```python
from build123d import *

# Parameters (mm, degrees)
EXTRUDE_1_DEPTH          = 2.5
SKETCH_5_R               = 0.6
CUT_EXTRUDE_1_DEPTH      = 19.036421485
CUT_EXTRUDE_START        = -2
SKETCH_5_3_R             = 1
CUT_EXTRUDE_2_DEPTH      = 1
REVOLVE_1_ANGLE          = 1
SKETCH_9_R               = 0.6
CUT_EXTRUDE_3_DEPTH      = 41.426698916
SKETCH_9_3_R             = 1
CUT_EXTRUDE_4_DEPTH      = 1
CUT_EXTRUDE_9_DEPTH      = 41.426698916
CUT_EXTRUDE_9_DEPTH_BACK = 41.426698916


with BuildPart() as part:
    # 草图4 → 凸台-拉伸1 (new body)
    with BuildSketch(Plane.XY):
        Polygon((8.5, -1.5), (17.75, -1.5), (17.75, -3.5), (-4.5, -3.5), (-4.5, -1.5), (-0.5, 0), (0, 0), (0, -1.5), (4, -1.5), (4, 0), (4.5, 0), align=None)
    extrude(amount=EXTRUDE_1_DEPTH)

    # 草图5 → 切除-拉伸1 (cut, through all)
    with BuildSketch(Plane(origin=(0, -1.5, 0), x_dir=(1, 0, 0), z_dir=(0, 1, 0))):
        with Locations(Location((2, -1.25, 0), (0, 0, 270))):
            Circle(SKETCH_5_R)
    extrude(amount=-CUT_EXTRUDE_1_DEPTH, mode=Mode.SUBTRACT)

    # 草图5<3> → 切除-拉伸2 (cut)
    with BuildSketch(Plane(origin=(0, -1.5, 0), x_dir=(1, 0, 0), z_dir=(0, 1, 0)).offset(CUT_EXTRUDE_START)):
        with Locations((2, -1.25)):
            Circle(SKETCH_5_3_R)
    extrude(amount=CUT_EXTRUDE_2_DEPTH, mode=Mode.SUBTRACT)

    # 镜向1: part across plane


with BuildPart() as part_1:
    add(part.part)
    add(part.part.mirror(Plane(origin=(17.75, 0, 2.5), x_dir=(0, 0, 1), z_dir=(1, 0, 0))))

    # 草图6 → 旋转1 (revolve)
    with BuildSketch(Plane.XY.offset(2.5)):
        Polygon((0, 0), (-0.5, 0), (-4.5, -1.5), (-4.5, -3.5), (40, -3.5), (40, -1.5), (36, 0), (35.5, 0), (35.5, -1.5), (31.5, -1.5), (31.5, 0), (31, 0), (27, -1.5), (8.5, -1.5), (4.5, 0), (4, 0), (4, -1.5), (0, -1.5), align=None)
    revolve(axis=Axis((-132.25, 94.8535776, 2.5), (0, -1, 0)), revolution_arc=REVOLVE_1_ANGLE)

    # 草图9 → 切除-拉伸3 (cut, through all)
    with BuildSketch(Plane(origin=(0, -1.5, 0), x_dir=(1, 0, 0), z_dir=(0, 1, 0))):
        with Locations(Location((1.994888171, -3.671537391, 0), (0, 0, 180))):
            Circle(SKETCH_9_R)
        with Locations(Location((33.493688748, -3.946423259, 0), (0, 0, 180))):
            Circle(SKETCH_9_R)
    extrude(amount=-CUT_EXTRUDE_3_DEPTH, mode=Mode.SUBTRACT)

    # 草图9<3> → 切除-拉伸4 (cut)
    with BuildSketch(Plane(origin=(0, -1.5, 0), x_dir=(1, 0, 0), z_dir=(0, 1, 0)).offset(CUT_EXTRUDE_START)):
        with Locations((1.994888171, -3.671537391)):
            Circle(SKETCH_9_3_R)
        with Locations((33.493688748, -3.946423259)):
            Circle(SKETCH_9_3_R)
    extrude(amount=CUT_EXTRUDE_4_DEPTH, mode=Mode.SUBTRACT)

    # 草图10 → 切除-拉伸9 (cut, two sides: drawn at the far end of the back side and taken through both)
    with BuildSketch(Plane(origin=(0, -1.5, 0), x_dir=(1, 0, 0), z_dir=(0, 1, 0)).offset(-CUT_EXTRUDE_9_DEPTH_BACK)):
        Polygon((27, -2.5), (27, -1.5), (24.5, -1.5), (25.667850814, -3.5), (20.832149186, -3.5), (22, -1.5), (17.164298372, -1.5), (18.332149186, -3.5), (13.496447557, -3.5), (14.664298372, -1.5), (9.828596743, -1.5), (10.996447557, -3.5), (8.496447557, -3.5), (8.5, -2.5), (-4.5, -2.5), (-4.5, 0), (40, 0), (40, -2.5), align=None)
    extrude(amount=CUT_EXTRUDE_9_DEPTH + CUT_EXTRUDE_9_DEPTH_BACK, mode=Mode.SUBTRACT)


solid = part_1.part
```
The model under review builds one solid part; all positions refer to its coordinate system, in mm. A direction names the side the tool comes from. Round coordinates to 2 decimals unless told otherwise and drop trailing zeros. Loops run counter-clockwise (first coordinate to the right, second up) from the corner with the lowest first, then second, coordinate; pieces in that order, holes last. Notation, with made-up numbers: (16, -13) - (58, -13) arc R14 ccw to (58, -7) - close; hole circle Ø11 at (58.25, 66). An arc over 180 degrees is marked (long way). Write each question's results on one line, items separated by ' | '. Start each with the question number.
Q1. Wall thickness on line 1 along X through (y, z) = (-2.75, 2.1); line 2 along X through (y, z) = (-1.7, 2.55); line 3 along Y through (x, z) = (23.5, 4.35): over which ranges is each line inside the solid? List them lowest first. Write a range as [from, to].
Q2. Tool access review of faces 1 (the flat face through (17.74, -2.514, 2.486)), 2 (the flat face through (2, -2, 2.5)), 3 (the flat face through (34, -2, 2.5)): name each direction out of +Z, -Z, +X, -X, +Y, -Y from which nothing blocks a thin tool from reaching the whole face with its end or side.
Q3. Take a section at C-C on y = -3. Give the boundary of the cut face in (x, z), plus the area to 3 significant figures.
Q4. Draft analysis for pull direction X (two halves, no side actions). For faces 4 (the flat face through (10, -3, 3.5)), 5 (the flat face through (2, -1.5, 4.5)), 6 (the cylindrical face through (39.994, -2.486, 3.982)), 7 (the flat face through (18, -3.5, 4)), state which applies: pulls with the +X half, pulls with the -X half, needs draft (parallel to the pull), parting line crosses it, or undercut.
Q5. Take a section at D-D on x = 35. Give the boundary of the cut face in (y, z).
Q6. Insertion check: P1, Ø1, axis at x = 16, y = -3, coming from the -Z side; P2, Ø0.5, axis at y = -3, z = 2, coming from the +X side; P3, Ø1.9, axis at x = 33.49, z = 3.95, coming from the -Y side. Each pin has a flat end and moves straight along its axis. Give the tip position at first contact, or say it passes through.
Q7. Take a section at B-B on x = 10.5. Give the boundary of the cut face in (y, z).
Q8. Take a section at A-A on y = -0.8. Give the boundary of the cut face in (x, z).
Data:
1) line 1: x = [10.18, 14.31], [17.51, 21.65], [24.85, 27] | line 2: x = [-4.5, 8.5], [10.44, 14.05], [17.78, 21.39], [25.11, 40] | line 3: y = [-3.5, -1.5]
2) face 1: +Y, -Y | face 2: -Z, -X, +Y, -Y | face 3: -Z, +X, +Y, -Y
3) outline: (-4.52, 4.73) arc R127.75 cw to (-4.5, 2.5) - (8.5, 2.5) - (8.5, 3.5) - (11, 3.5) - (9.83, 1.5) - (14.66, 1.5) - (13.5, 3.5) - (18.33, 3.5) - (17.16, 1.5) - (22, 1.5) - (20.83, 3.5) - (25.67, 3.5) - (24.5, 1.5) - (27, 1.5) - (27, 2.5) - (40, 2.5) arc R172.25 ccw to (39.97, 5.51) - close; hole circle Ø2 at (1.99, 3.67); hole circle Ø2 at (33.49, 3.95) | area: 110 mm²
4) face 4: undercut | face 5: undercut | face 6: pulls with the +X half | face 7: needs draft
5) outline: (-3.5, 2.5) - (-1.5, 2.5) - (-1.5, 5.42) - (-3.5, 5.42) - close
6) P1: stops at z = 3.5 | P2: stops at x = 27 | P3: stops at y = -2.5
7) outline: (-3.5, 1.5) - (-1.5, 1.5) - (-1.5, 2.65) - (-3.5, 2.65) - close; (-3.5, 3.5) - (-1.5, 3.5) - (-1.5, 4.99) - (-3.5, 4.99) - close
8) outline: (-2.65, 4.76) arc R129.62 cw to (-2.63, 2.5) - (0, 2.5) arc R132.25 ccw to (-0.02, 4.81) - close; (3.98, 4.88) arc R136.25 cw to (4, 2.5) - (6.63, 2.5) arc R138.88 ccw to (6.61, 4.92) - close; (28.84, 5.31) arc R161.12 cw to (28.87, 2.5) - (31.5, 2.5) arc R163.75 ccw to (31.48, 5.36) - close; (35.47, 5.43) arc R167.75 cw to (35.5, 2.5) - (38.13, 2.5) arc R170.38 ccw to (38.11, 5.47) - close
